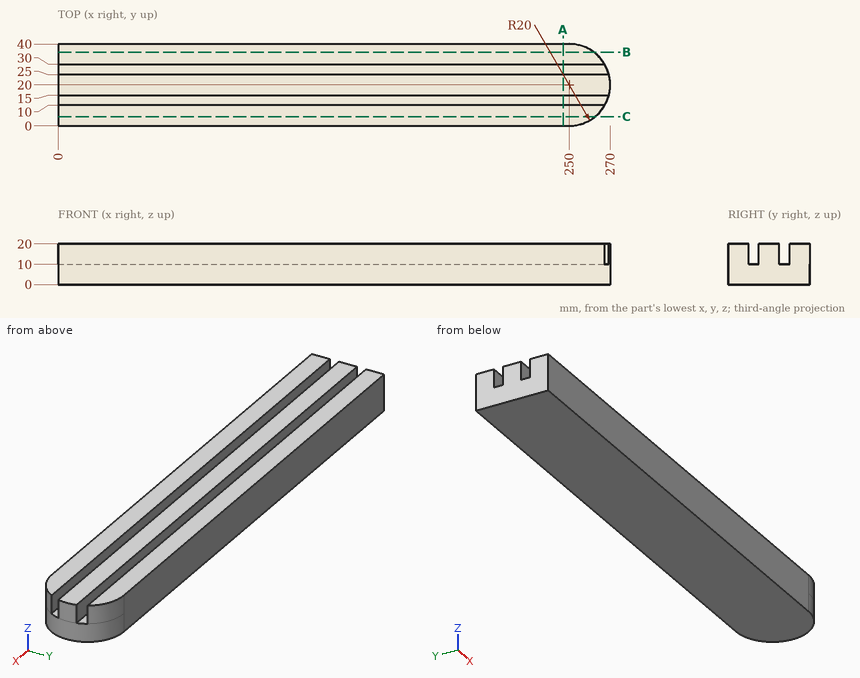
Study the drawing (mm; zero at the part's minimum x, y, z) and answer. Coordinates: 2 decimals unless noted, no trailing zeros. Loops run counter-clockwise (first coordinate to the right, second up) from the corner with the lowest first, then second, coordinate; pieces in that order, holes last. Notation, with made-up numbers: M -6.75,47 L 13.25,47 A27 cw 13.25,82 Z; hole C 52,-25.5 d6. An arc over 180 degrees is marked long. Answer as a JSON object with one key per item and string values. Group by question number.
Item 1: Consider L1, parallel to Y at x = 28.5, z = 12.5; L2, parallel to Z at x = 33.5, y = 29.5; L3, parallel to X at y = 30.5, z = 2.5. Determine where each line is inside the solid, lowest interval first.
Item 2: Section C-C (y = 4.5) is taken. Write down the section's boundary in (x, z), and give its area (3 significant figures).
Item 3: Section B-B (y = 36) is taken. Write down the section's boundary in (x, z).
Item 4: Each of these flat-tipped pins is pushed along its axis until it touches: P1, Ø6, axis at x = 220.5, y = 35.5, coming from the -Z side; P2, Ø10, axis at y = 29.5, z = 17, coming from the +X side; P3, Ø12, axis at y = 19, z = 14.5, coming from the +X side; P4, Ø12, axis at y = 36, z = 7.5, coming from the +X side. Where does it stop, or does it pass through?
Item 5: Section A-A (x = 247) is taken. Write down the section's boundary in (y, z).
Solved:
{
 "1": {"L1": "y = 0 to 10, 15 to 25, 30 to 40", "L2": "z = 0 to 10", "L3": "x = 0 to 267.02"},
 "2": {"outline": "M 0,0 L 262.64,0 L 262.64,20 L 0,20 Z", "area": "5,250 mm2"},
 "3": {"outline": "M 0,0 L 262,0 L 262,20 L 0,20 Z"},
 "4": {"P1": "stops at z = 0", "P2": "stops at x = 269.49", "P3": "stops at x = 270", "P4": "stops at x = 267.32"},
 "5": {"outline": "M 0,0 L 40,0 L 40,20 L 30,20 L 30,10 L 25,10 L 25,20 L 15,20 L 15,10 L 10,10 L 10,20 L 0,20 Z"}
}
